from build123d import *

# Parameters (mm, degrees)
ESQUISSE1_R             = 2
ESQUISSE1_R_2           = 3.5
BASE_EXTRUSION_DEPTH    = 2.5
ESQUISSE2_R             = 0.75
ENL_V_MAT_EXTRU_1_DEPTH = 10


with BuildPart() as part:
    # Esquisse1 → Base-Extrusion (new, symmetric)
    with BuildSketch(Plane.XY):
        with BuildLine():
            Line((4.604526211, -4.009780949), (24.808694688, -3.009780949))
            ThreePointArc((24.808694688, -3.009780949), (26.64302969, -3.130458818), (28.401389492, -3.666666667))
            ThreePointArc((28.401389492, -3.666666667), (34, 0), (28.401389492, 3.666666667))
            ThreePointArc((28.401389492, 3.666666667), (26.64302969, 3.130458818), (24.808694688, 3.009780949))
            Line((24.808694688, 3.009780949), (4.604526211, 4.009780949))
            ThreePointArc((4.604526211, 4.009780949), (3.237594273, 4.196543967), (1.923076923, 4.615384615))
            ThreePointArc((1.923076923, 4.615384615), (-5, 0), (1.923076923, -4.615384615))
            ThreePointArc((1.923076923, -4.615384615), (3.237594273, -4.196543967), (4.604526211, -4.009780949))
        make_face()
        with Locations((30, 0)):
            Circle(ESQUISSE1_R, mode=Mode.SUBTRACT)
        Circle(ESQUISSE1_R_2, mode=Mode.SUBTRACT)
    extrude(amount=BASE_EXTRUSION_DEPTH, both=True)

    # Esquisse2 → Enlèv. mat.-Extru.1 (cut, symmetric)
    with BuildSketch(Plane(origin=(0, 0, 0), x_dir=(1, 0, 0), z_dir=(0, 1, 0))):
        with Locations(Location((0, 0, 0), (0, 0, 270))):
            Circle(ESQUISSE2_R)
        with BuildLine():
            Line((5, 6.563022401), (25, 6.563022401))
            Line((25, 6.563022401), (25, 3.5))
            ThreePointArc((25, 3.5), (24.414213562, 2.085786438), (23, 1.5))
            Line((23, 1.5), (7, 1.5))
            ThreePointArc((7, 1.5), (5.585786438, 2.085786438), (5, 3.5))
            Line((5, 3.5), (5, 6.563022401))
        make_face()
        with BuildLine():
            Line((5, -5.954530257), (25, -5.954530257))
            Line((25, -5.954530257), (25, -3.5))
            ThreePointArc((25, -3.5), (24.414213562, -2.085786438), (23, -1.5))
            Line((23, -1.5), (7, -1.5))
            ThreePointArc((7, -1.5), (5.585786438, -2.085786438), (5, -3.5))
            Line((5, -3.5), (5, -5.954530257))
        make_face()
    extrude(amount=ENL_V_MAT_EXTRU_1_DEPTH, both=True, mode=Mode.SUBTRACT)


solid = part.part
Geometry: final body of the model. Coordinates: model frame, mm. A direction names the side the tool comes from. Coordinates: 2 decimals unless noted, no trailing zeros. Loops run counter-clockwise (first coordinate to the right, second up) from the corner with the lowest first, then second, coordinate; pieces in that order, holes last. Notation, with made-up numbers: (10, 89) - (64, 89) arc R31 ccw to (64, 115) - close; hole circle Ø6 at (10, -30). An arc over 180 degrees is marked (long way). Put each result on its own line as item: value. Start each with the question number.
Q1. Line query: line 1 (Y direction, x = 30, z = 0.5); line 2 (Z direction, x = 0, y = 4.5); line 3 (X direction, y = -1, z = -0.9). Output: solid intervals per line, ascending.
Q2. Cut plane C-C, the plane x = 0. Return loops of the section in (y, z).
Q3. Set-up query: faces 4 (the cylindrical face through (24.013, -0.043, -1.775)), 5 (the flat face through (14.565, -3.517, 0.035)), 6 (the cylindrical face through (24.013, 0.043, 1.775)). Return all of +Z, -Z, +X, -X, +Y, -Y with unobstructed straight access to the full face (end or side cutting, diameter ignored); none if empty.
Q4. Cut plane B-B, the plane z = -0.4. Return loops of the section in (x, y).
Q5. Pin query (flat end, axial travel): pin 1 Ø1 at (x, z) = (25, 1.5) entering from -Y; pin 2 Ø4 at (x, y) = (12.5, -1) entering from +Z; pin 3 Ø1.5 at (x, z) = (7.5, -0.5) entering from -Y. Return the tip coordinate at first contact, or that it passes through.
Q6. Cut plane A-A, the plane x = 30. Return loops of the section in (y, z), and give its area (3 significant figures).
Q7. Pull-direction query (X, two-part tool) for faces 1 (the flat face through (14.848, 3.503, 0.035)), 2 (the cylindrical face through (3.22, -4.2, 0.04)), 3 (the flat face through (27, 0, -2.5)); classes: released by +X, released by -X, zero draft, split by the parting line, or undercut.
Q8. Cut plane D-D, the plane y = 2.5. Return loops of the section in (x, z), and give its area (3 significant figures).
Filled sheet:
1. line 1: -4 to -2, 2 to 4
1. line 2: -2.5 to -0.75, 0.75 to 2.5
1. line 3: -4.9 to -3.35, 3.35 to 28.27, 31.73 to 33.87
2. outline: (-5, -2.5) - (-3.5, -2.5) - (-3.5, -0.75) - (-5, -0.75) - close; (-5, 0.75) - (-3.5, 0.75) - (-3.5, 2.5) - (-5, 2.5) - close; (3.5, -2.5) - (5, -2.5) - (5, -0.75) - (3.5, -0.75) - close; (3.5, 0.75) - (5, 0.75) - (5, 2.5) - (3.5, 2.5) - close
3. face 4: -Z, +Y, -Y
3. face 5: +Z, -Z, -Y
3. face 6: +Z, +Y, -Y
4. outline: (-0.63, -4.96) - (-0.63, -3.44) arc R3.5 cw to (-0.63, 3.44) - (-0.63, 4.96) arc R5 ccw to start; (0.63, -4.96) arc R5 ccw to (1.92, -4.62) arc R8 cw to (4.6, -4.01) - (24.81, -3.01) arc R8 cw to (28.4, -3.67) arc R4 ccw (long way) to (28.4, 3.67) arc R8 cw to (24.81, 3.01) - (4.6, 4.01) arc R8 cw to (1.92, 4.62) arc R5 ccw to (0.63, 4.96) - (0.63, 3.44) arc R3.5 cw to (0.63, -3.44) - close; hole circle Ø4 at (30, 0)
5. pin 1: y = -3.03
5. pin 2: z = 1.5
5. pin 3: y = -3.9
6. outline: (-4, -2.5) - (-2, -2.5) - (-2, 2.5) - (-4, 2.5) - close; (2, -2.5) - (4, -2.5) - (4, 2.5) - (2, 2.5) - close
6. area: 20.0 mm²
7. face 1: undercut
7. face 2: released by +X
7. face 3: zero draft
8. outline: (-4.33, -2.5) - (-2.45, -2.5) - (-2.45, 2.5) - (-4.33, 2.5) - close; (2.45, -2.5) - (5.27, -2.5) arc R2 cw to (7, -1.5) - (23, -1.5) arc R2 cw to (24.73, -2.5) - (33.12, -2.5) - (33.12, 2.5) - (24.73, 2.5) arc R2 cw to (23, 1.5) - (7, 1.5) arc R2 cw to (5.27, 2.5) - (2.45, 2.5) - close
8. area: 126 mm²
